Answer from the drawing. Dimensions are ordinates in mm from the lowest x, y and z of the part. Give positions to 0.01 mm unless a question says otherwise; leave off trailing zeros. Order: outer loops, then holes, each group sorted by start corner. A loop starts at its lowest first (then second) coordinate and runs counter-clockwise, first axis right, second up.
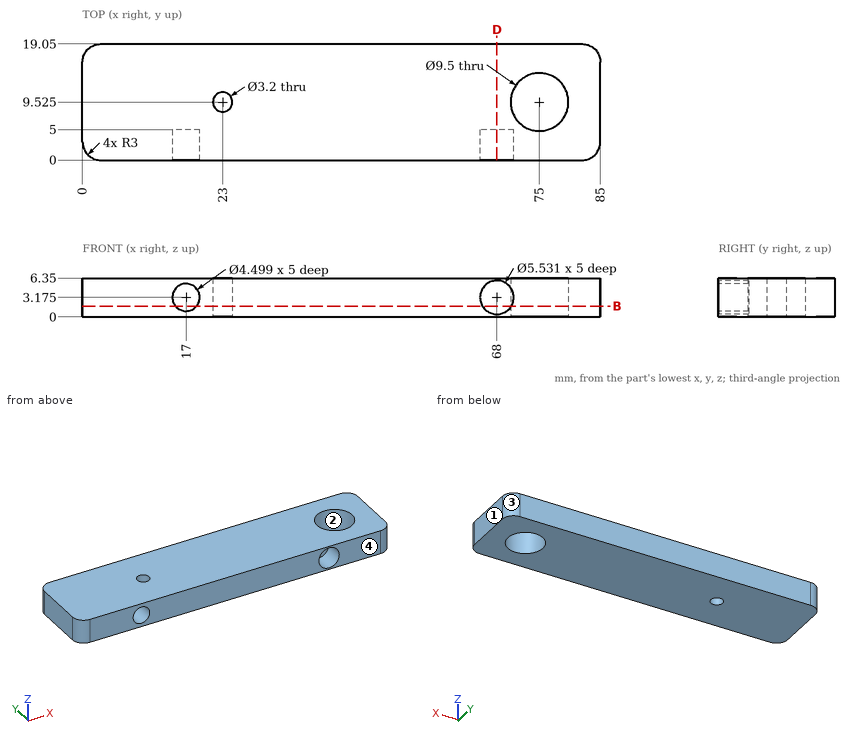
1) The part is cut by section B-B on z = 1.75. Count the separate pieces of the cut face and the enclosed holes in it, and give its area (3 significant figures).
Final values:
separate pieces: 1
enclosed holes: 2
area: 1,490 mm2
2) For a pull along Y with two mould halves and no side action, classify the marked faces 1, 2, 3 and 4 as released by +Y, released by -Y, zero draft, split by the parting line, or undercut.
Final values:
face 1: zero draft
face 2: undercut
face 3: released by +Y
face 4: released by -Y
3) Given pin 1 (3 mm diameter, centred on x = 23, y = 9.525, fed in from +Z); pin 2 (1.7 mm diameter, centred on x = 68.5, z = 4, fed in from -Y), each flat-ended and moving along its own axis, determine where each tip first touches the part or whether it passes through.
Final values:
pin 1: passes through
pin 2: stops at y = 5
4) The part is cut by section D-D on x = 68. Determine the outline of the cut face in (y, z).
Final values:
outline: (0, 0) - (19.05, 0) - (19.05, 6.35) - (0, 6.35) - (0, 5.94) - (5, 5.94) - (5, 0.41) - (0, 0.41) - close
5) Consider L1, parallel to Z at x = 68, y = 3.65; L2, parallel to Z at x = 17, y = 2.6; L3, parallel to X at y = 10.25, z = 4 (1 decimal). Determine where each line is inside the solid, lowest interval first.
Final values:
L1: z = 0 to 0.41, 5.94 to 6.35
L2: z = 0 to 0.93, 5.42 to 6.35
L3: x = 0 to 21.6, 24.4 to 70.3, 79.7 to 85
